Source: CAD feature listing. Evaluate the final solid. Frame: model axes, mm. A direction names the side the tool comes from. Round coordinates to 2 decimals unless told otherwise and drop trailing zeros. Order: outer loops, then holes, each group sorted by start corner. A loop starts at its lowest first (then second) coordinate and runs counter-clockwise, first axis right, second up. Notation, with made-up numbers: (-13.5, 56) -> (11.5, 56) arc R13 cw to (11.5, 78) -> close; hole circle Ø10 at (88.5, -27.5). An arc over 180 degrees is marked (long way). Answer as CSV lines item,"result". Start each with the question number.
(1) Set-up query: faces 1 (the flat face through (0, 0, -10)), 2 (the flat face through (-1.25, 0, 2)), 3 (the cylindrical face through (-1.45, 0.06, -4.93)). Return all of +Z, -Z, +X, -X, +Y, -Y with unobstructed straight access to the full face (end or side cutting, diameter ignored); none if empty.
(2) Section query C-C (z = -1). Output: boundary loops of the cut face in (x, y), plus the area to 3 significant figures.
(3) Section query D-D (x = -2.2). Output: boundary loops of the cut face in (y, z).
(4) Pull-direction query (Y, two-part tool) for faces 4 (the flat face through (1.2, -1.2, 0)), 5 (the cylindrical face through (-0.596, -2.685, 1.479)), 6 (the flat face through (0, 0, 1.05)); classes: +Y half, -Y half, draft (parallel to the pull), parting line (faces both ways), or undercut.
(5) Section query B-B (x = 0.7). Output: boundary loops of the cut face in (y, z), plus the area to 3 significant figures.
(6) Contact query for flat-ended pins moving along their axis: P1, Ø2, axis at y = -1.5, z = -2.5, coming from the -X side; P2, Ø2, axis at y = 1.5, z = 1.5, coming from the +X side; P3, Ø2, axis at x = 1.5, y = -2, coming from the -Z side. Output: stop coordinate, or through.
(7) Line query: line 1 along Y through (x, z) = (0.7, 2); line 2 along Z through (x, y) = (-0.2, 0.65); line 3 along X through (y, z) = (-0.95, 1.75). Output: solid intervals per line, ascending. Write a range as from..to.
(8) Section query A-A (y = 0). Output: boundary loops of the cut face in (x, z), plus the area to 3 significant figures.
```python
from build123d import *

# Parameters (mm, degrees)
SKETCH_1_R                     = 1.45
SHANK_THREADS_SIMPLIFIED_DEPTH = 10
SKETCH_2_R                     = 2.75
SOCKET_HEAD_DEPTH              = 3
HEX_SOCKET_DEPTH               = 1.95


with BuildPart() as part:
    # 草图1 → Shank_threads_simplified (new body)
    with BuildSketch(Plane.XY):
        Circle(SKETCH_1_R)
    extrude(amount=-SHANK_THREADS_SIMPLIFIED_DEPTH)

    # 草图2 → Socket_head (add)
    with BuildSketch(Plane.XY):
        Circle(SKETCH_2_R)
    extrude(amount=SOCKET_HEAD_DEPTH)

    # 草图3 → Hex_socket (cut)
    with BuildSketch(Plane.XY.offset(3)):
        Polygon((1.25, 0.721687836), (0, 1.443375673), (-1.25, 0.721687836), (-1.25, -0.721687836), (0, -1.443375673), (1.25, -0.721687836), align=None)
    extrude(amount=-HEX_SOCKET_DEPTH, mode=Mode.SUBTRACT)


solid = part.part
```
Answer block:
1,face 1,"-Z, +X, -X, +Y, -Y"
1,face 2,"+Z"
1,face 3,"-Z"
2,outline,"circle Ø2.9 at (0, 0)"
2,area,"6.61 mm2"
3,outline,"(-1.65, 0) -> (1.65, 0) -> (1.65, 3) -> (-1.65, 3) -> close"
4,face 4,"draft"
4,face 5,"parting line"
4,face 6,"undercut"
5,outline,"(-2.66, 0) -> (-1.27, 0) -> (-1.27, -10) -> (1.27, -10) -> (1.27, 0) -> (2.66, 0) -> (2.66, 3) -> (1.04, 3) -> (1.04, 1.05) -> (-1.04, 1.05) -> (-1.04, 3) -> (-2.66, 3) -> close"
5,area,"37.3 mm2"
6,P1,"x = -1.36"
6,P2,"x = 2.7"
6,P3,"z = 0"
7,line 1,"-2.66..-1.04, 1.04..2.66"
7,line 2,"-10..1.05"
7,line 3,"-2.58..-0.85, 0.85..2.58"
8,outline,"(-2.75, 0) -> (-1.45, 0) -> (-1.45, -10) -> (1.45, -10) -> (1.45, 0) -> (2.75, 0) -> (2.75, 3) -> (1.25, 3) -> (1.25, 1.05) -> (-1.25, 1.05) -> (-1.25, 3) -> (-2.75, 3) -> close"
8,area,"40.6 mm2"
